Can you work these out from the model? Positions are in its coordinate system, mm. Face numbers are marked on the shaded views. A direction names the side the tool comes from. Give positions to 0.01 mm unless a question says otherwise; leave off trailing zeros. Loops run counter-clockwise (first coordinate to the right, second up) from the corner with the lowest first, then second, coordinate; pieces in that order, holes last. Notation, with made-up numbers: M 41,67 L 88,67 A18 cw 88,90 Z; hole C -5.75,50 d10. An arc over 180 degrees is marked long. Use CSV: the item, a comma, the result in double quotes.
from build123d import *

# Parameters (mm, degrees)
SCHIZZO2_W                          = 20
SCHIZZO2_H                          = 20
SCHIZZO2_R                          = 0.15
ESTRUSIONE_ESTRUSIONE1_DEPTH        = 10
SCHIZZO3_R                          = 4
SCHIZZO3_R_2                        = 1.75
ESTRUSIONE_SOTTILE1_DEPTH           = 13
TAGLIO_ESTRUSIONE1_REACH            = 34.078
SCHIZZO4_R                          = 3
SCHIZZO4_R_2                        = 1.15
FORO_FILETTATO_M6X1_0_1_D           = 5
FORO_FILETTATO_M6X1_0_1_DEPTH       = 12
FORO_FILETTATO_M6X1_0_1_CSINK_D     = 6.05
FORO_FILETTATO_M6X1_0_1_CSINK_ANGLE = 90
FORO_FILETTATO_M6X1_0_1_TIP         = 1.502151548
SCHIZZO8_R                          = 13
SCHIZZO8_R_2                        = 3
TAGLIO_ESTRUSIONE_SOTTILE1_DEPTH    = 3


with BuildPart() as part:
    # Schizzo1 → Rivoluzione1 (revolve)
    with BuildSketch(Plane.XY, mode=Mode.PRIVATE) as rivoluzione1_sk:
        Polygon((-0.15, 0), (-0.15, -5), (-0.5, -5), (-3, -2), (-3, 0), align=None)
    revolve(rivoluzione1_sk.sketch.rotate(Axis((0, -26.528171736, 0), (0, 1, 0)), 270), axis=Axis((0, -26.528171736, 0), (0, 1, 0)))

    # Schizzo2 → Estrusione-Estrusione1 (add)
    with BuildSketch(Plane(origin=(0, 0, 0), x_dir=(1, 0, 0), z_dir=(0, 1, 0))):
        Rectangle(SCHIZZO2_W, SCHIZZO2_H)
        with Locations(Location((0, 0, 0), (0, 0, 90))):
            Circle(SCHIZZO2_R, mode=Mode.SUBTRACT)
    extrude(amount=ESTRUSIONE_ESTRUSIONE1_DEPTH)

    # Schizzo3 → Estrusione-Sottile1 (add)
    with BuildSketch(Plane(origin=(0, 10, 0), x_dir=(1, 0, 0), z_dir=(0, 1, 0))):
        Circle(SCHIZZO3_R)
        Circle(SCHIZZO3_R_2, mode=Mode.SUBTRACT)
    extrude(amount=ESTRUSIONE_SOTTILE1_DEPTH)

    # Schizzo4 → Taglio-Estrusione1 (cut, up to next)
    with BuildSketch(Plane.XY.offset(10), mode=Mode.PRIVATE) as taglio_estrusione1_sk1:
        with Locations((-6, 5)):
            Circle(SCHIZZO4_R)
    taglio_estrusione1_tool1 = extrude(taglio_estrusione1_sk1.sketch, amount=-TAGLIO_ESTRUSIONE1_REACH, mode=Mode.PRIVATE) & part.part
    # Schizzo4 → Taglio-Estrusione1 (cut, up to next)
    with BuildSketch(Plane.XY.offset(10), mode=Mode.PRIVATE) as taglio_estrusione1_sk2:
        with Locations((6, 5)):
            Circle(SCHIZZO4_R_2)
    taglio_estrusione1_tool2 = extrude(taglio_estrusione1_sk2.sketch, amount=-TAGLIO_ESTRUSIONE1_REACH, mode=Mode.PRIVATE) & part.part
    add(taglio_estrusione1_tool1.solids().sort_by_distance((-6, 5, 10))[0], mode=Mode.SUBTRACT)
    add(taglio_estrusione1_tool2.solids().sort_by_distance((6, 5, 10))[0], mode=Mode.SUBTRACT)

    # Foro filettato M6x1.0-1
    with Locations(Plane(origin=(0, 0, -10), x_dir=(-1, 0, 0), z_dir=(0, 0, -1))):
        with Locations((-6, 5)):
            CounterSinkHole(FORO_FILETTATO_M6X1_0_1_D / 2, FORO_FILETTATO_M6X1_0_1_CSINK_D / 2, depth=FORO_FILETTATO_M6X1_0_1_DEPTH, counter_sink_angle=FORO_FILETTATO_M6X1_0_1_CSINK_ANGLE)
            with Locations((0, 0, -(FORO_FILETTATO_M6X1_0_1_DEPTH + FORO_FILETTATO_M6X1_0_1_TIP / 2))):  # 118° drill point
                Cone(0, FORO_FILETTATO_M6X1_0_1_D / 2, FORO_FILETTATO_M6X1_0_1_TIP, mode=Mode.SUBTRACT)

    # Schizzo8 → Taglio-Estrusione-Sottile1 (cut)
    with BuildSketch(Plane(origin=(0, 23, 0), x_dir=(1, 0, 0), z_dir=(0, 1, 0))):
        Circle(SCHIZZO8_R)
        Circle(SCHIZZO8_R_2, mode=Mode.SUBTRACT)
    extrude(amount=-TAGLIO_ESTRUSIONE_SOTTILE1_DEPTH, mode=Mode.SUBTRACT)


solid = part.part
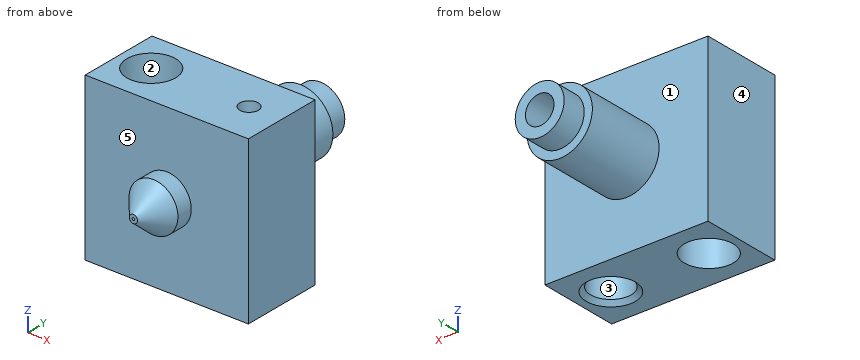
Q1. I want a section at C-C, the plane z = 7.25. Please give me the cut outline in (x, y).
Model answer:
outline,"M -10,0 L 10,0 L 10,10 L -10,10 Z; hole C -6,5 d6; hole C 6,5 d2.3"
Q2. For the marked faces 1 and 2, which set-ups out of +Z, -Z, +X, -X, +Y, -Y let a thin tool reach every point of the face, with its end or its side?
Model answer:
face 1,"+Y"
face 2,"+Z, -Z"
Q3. I want a section at D-D, the plane x = 6. Please give me the cut outline in (y, z) (3 decimals), then the cut area to 3 significant figures.
Model answer:
outline,"M 0,-10 L 1.975,-10 L 2.5,-9.475 L 2.5,2 L 3.85,2.811 L 3.85,10 L 0,10 Z; M 6.15,2.811 L 7.5,2 L 7.5,-9.475 L 8.025,-10 L 10,-10 L 10,10 L 6.15,10 Z"
area,"120 mm2"
Q4. I want a section at A-A, the plane y = 5. Please give me the cut outline in (x, z) (3 decimals).
Model answer:
outline,"M -10,-10 L -9,-10 L -9,10 L -10,10 Z; M -3,-10 L 2.975,-10 L 3.5,-9.475 L 3.5,2 L 4.85,2.811 L 4.85,10 L -3,10 Z; M 7.15,2.811 L 8.5,2 L 8.5,-9.475 L 9.025,-10 L 10,-10 L 10,10 L 7.15,10 Z; hole C 0,0 d0.3"
Q5. If we mould it in two halves opening along Y, with no side actions, what happens to the marked faces 3, 4 and 5? For each: released by +Y, released by -Y, zero draft, split by the parting line, or undercut.
Model answer:
face 3,"undercut"
face 4,"zero draft"
face 5,"released by -Y"
Q6. Please list where these lines run through material, in increasing order: L1, parallel to X at y = 2.25, z = 0; L2, parallel to Z at x = 0, y = 14.5; L3, parallel to Y at x = -6, z = 0. Write a range as from..to.
Model answer:
L1,"-10..-7.2, -4.8..-0.15, 0.15..10"
L2,"-4..-1.75, 1.75..4"
L3,"0..2, 8..10"
Q7. I want a section at B-B, the plane x = -6. Please give me the cut outline in (y, z), then the cut area to 3 significant figures.
Model answer:
outline,"M 0,-10 L 2,-10 L 2,10 L 0,10 Z; M 8,-10 L 10,-10 L 10,10 L 8,10 Z"
area,"80.0 mm2"
Q8. I'm going to push flat-ended pins straight in: P1, Ø5, axis at x = -3.5, z = 4, coming from the -Y side; P2, Ø1.5, axis at x = -4.5, z = 7.5, coming from the -Y side; P3, Ø5, axis at x = 2.5, y = 18.5, coming from the +Z side. Where does each tip first touch, or does it pass through?
Model answer:
P1,"y = -2.22"
P2,"y = 0"
P3,"z = 4"
